For this review, take the finished solid that the model builds, in its own axes (mm). Round coordinates to 2 decimals unless told otherwise and drop trailing zeros. Loops run counter-clockwise (first coordinate to the right, second up) from the corner with the lowest first, then second, coordinate; pieces in that order, holes last. Notation, with made-up numbers: (57.25, -35) -> (70.25, -35) arc R19 ccw to (70.25, -13) -> close; hole circle Ø10 at (31, -20.5). An arc over 180 degrees is marked (long way). Use one line per item in the form item = value. Start each with the question number.
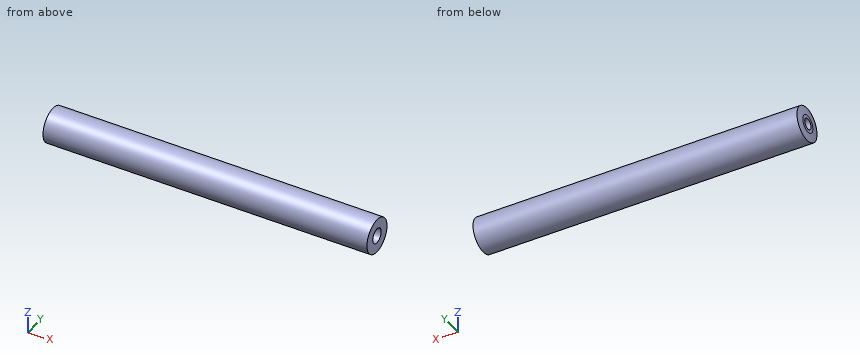
from build123d import *

# Parameters (mm, degrees)
F3_D     = 5
F3_DEPTH = 15
F3_TIP   = 1.5021515476
F5_D     = 6.8
F5_DEPTH = 20
F5_TIP   = 2.0429261047


with BuildPart() as f1:
    # F0 (on Front) → F1 (revolve)
    with BuildSketch(Plane.XZ):
        with BuildLine():
            Line((-75.2020410289, 0), (75.2020410289, 0))
            Line((75.2020410289, 0), (75.2020410289, 8))
            Line((75.2020410289, 8), (-74.7979589711, 8))
            ThreePointArc((-74.7979589711, 8), (-75.100764089, 6.0101792401), (-75.2020410289, 4))
            Line((-75.2020410289, 4), (-75.2020410289, 0))
        make_face()
    revolve(axis=Axis((-20.4167328775, 0, 0), (1, 0, 0)))

    # F3
    with Locations(Plane(origin=(-75.2020410289, 0, 0), x_dir=(0, -1, 0), z_dir=(-1, 0, 0))):
        with Locations((0, 0)):
            Hole(F3_D / 2, depth=F3_DEPTH)
            with Locations((0, 0, -(F3_DEPTH + F3_TIP / 2))):  # 118° drill point
                Cone(0, F3_D / 2, F3_TIP, mode=Mode.SUBTRACT)

    # F5
    with Locations(Plane.YZ.offset(75.2020410289)):
        with Locations((0, 0)):
            Hole(F5_D / 2, depth=F5_DEPTH)
            with Locations((0, 0, -(F5_DEPTH + F5_TIP / 2))):  # 118° drill point
                Cone(0, F5_D / 2, F5_TIP, mode=Mode.SUBTRACT)


solid = f1.part
Item 1: Wall thickness on line 1 (Y direction, x = -68, z = 0); line 2 (Z direction, x = 68.75, y = 0): over which ranges is each line inside the solid? List them lowest first.
Item 2: Take a section at A-A on x = -19.5. Give the boundary of the cut face in (y, z), plus the area to 3 significant figures.
Item 3: For P1, Ø1, axis at x = -56.5, y = 1.5, coming from the +Z side; P2, Ø4.5, axis at y = 0, z = 0, coming from the +X side; P3, Ø4, axis at x = -38.5, y = 2, coming from the +Z side; P4, Ø5.5, axis at y = 0, z = 0, coming from the +X side, all flat-tipped, find the tip position at first contact; note any pin that passes through.
Results:
q1.line_1 = -8 to -2.5, 2.5 to 8
q1.line_2 = -8 to -3.4, 3.4 to 8
q2.outline = circle Ø16 at (0, 0)
q2.area = 201 mm2
q3.P1 = 7.94
q3.P2 = 54.51
q3.P3 = 8
q3.P4 = 54.81
